Geometry: final body of the model. Coordinates: model frame, mm. Give positions to 0.01 mm unless a question says otherwise; leave off trailing zeros. Loops run counter-clockwise (first coordinate to the right, second up) from the corner with the lowest first, then second, coordinate; pieces in that order, holes last.
1. First-contact query: P1, Ø3, axis at x = 219.5, z = -7.5, coming from the +Y side; P2, Ø1, axis at x = 309, y = 6, coming from the -Z side; P3, Ø6, axis at x = 119, z = -3, coming from the -Y side. Flat tips, straight axial feed; report the tip coordinate or a pass-through.
2. Section A-A, the plane x = 151.5. Output: boundary loops of the cut face in (y, z), then the cut area to 4 significant figures.
3. Material intervals for line 1 along Y through (x, z) = (277.5, -8); line 2 along Z through (x, y) = (326, 11); line 3 along X through (y, z) = (1.25, -7), sorted ascending.
4. Section B-B, the plane z = -10.5. Output: boundary loops of the cut face in (x, y), then the cut area to 3 significant figures.
5. Section C-C, the plane y = 8.5. Output: boundary loops of the cut face in (x, z), then the cut area to 4 significant figures.
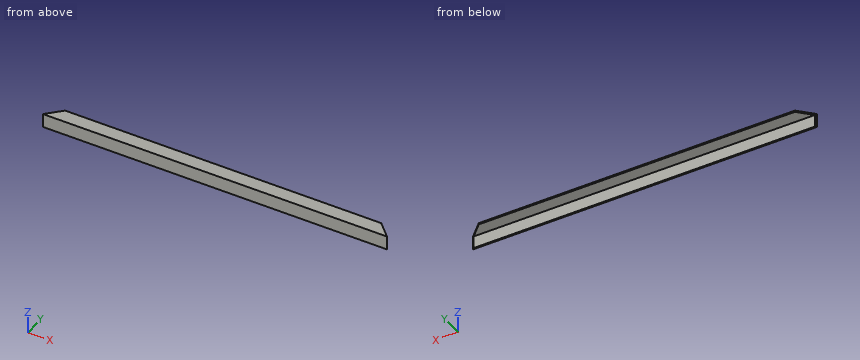
from build123d import *

# Parameters (mm, degrees)
EXTRUDE_1_DEPTH     = 370
CUT_EXTRUDE_1_DEPTH = 16


with BuildPart() as part:
    # Эскиз1 → Бобышка-Вытянуть1 (new body)
    with BuildSketch(Plane(origin=(0, 0, 0), x_dir=(0, 0, -1), z_dir=(1, 0, 0))):
        Polygon((0, 0), (0, 15), (1.5, 15), (1.5, 1.5), (15, 1.5), (15, 0), align=None)
    extrude(amount=EXTRUDE_1_DEPTH)

    # Эскиз2 → Вырез-Вытянуть1 (cut, through all)
    with BuildSketch(Plane.XY):
        Polygon((0, 0), (22.757405311, 22.757405311), (0, 22.757405311), align=None)
    cut_extrude_1 = extrude(amount=-CUT_EXTRUDE_1_DEPTH, mode=Mode.SUBTRACT)

    # Зеркальное отражение1: Вырез-Вытянуть1 across plane
    add(cut_extrude_1.mirror(Plane.ZY.offset(-185)), mode=Mode.SUBTRACT)


solid = part.part
Answers below:
1. P1: stops at y = 1.5
1. P2: stops at z = -1.5
1. P3: stops at y = 0
2. outline: (0, -15) - (1.5, -15) - (1.5, -1.5) - (15, -1.5) - (15, 0) - (0, 0) - close
2. area: 42.75 mm2
3. line 1: y = 0 to 1.5
3. line 2: z = -1.5 to 0
3. line 3: x = 1.25 to 368.75
4. outline: (0, 0) - (370, 0) - (368.5, 1.5) - (1.5, 1.5) - close
4. area: 553 mm2
5. outline: (8.5, -1.5) - (361.5, -1.5) - (361.5, 0) - (8.5, 0) - close
5. area: 529.5 mm2
